Read the model definition and answer for the solid it produces. Units are mm, in the model's axes. Give positions to 0.01 mm unless a question says otherwise; leave off trailing zeros. Order: outer loops, then holes, each group sorted by start corner. A loop starts at its lowest first (then second) coordinate and runs counter-clockwise, first axis right, second up. Notation, with made-up numbers: (82.5, 85.5) - (113.5, 85.5) arc R16 cw to (113.5, 109.5) - close; hole circle Ø8 at (40.25, 10.5). An arc over 180 degrees is marked (long way). Write item = value, one per line.
```python
from build123d import *

# Parameters (mm, degrees)
SKETCH_1_R      = 1.5
SKETCH_1_R_2    = 2
EXTRUDE_1_DEPTH = 3
FILLET_1_R      = 2


with BuildPart() as part:
    # 草图1 → 凸台-拉伸1 (new body)
    with BuildSketch(Plane(origin=(0, 0, 0), x_dir=(1, 0, 0), z_dir=(0, 1, 0))):
        with BuildLine():
            Line((30, -10.5), (20.838488019, -10.5))
            ThreePointArc((20.838488019, -10.5), (19.128387303, -10.801536896), (17.624549971, -11.669777784))
            Line((17.624549971, -11.669777784), (8.432016653, -19.383229101))
            ThreePointArc((8.432016653, -19.383229101), (7.315827683, -20.713451316), (6.721915937, -22.345210428))
            Line((6.721915937, -22.345210428), (2.526313412, -46.139654751))
            Line((2.526313412, -46.139654751), (-18.154649402, -42.49304302))
            Line((-18.154649402, -42.49304302), (-10.267627346, 2.236481777))
            ThreePointArc((-10.267627346, 2.236481777), (-6.847425912, 8.160444431), (-0.419549816, 10.5))
            Line((-0.419549816, 10.5), (30, 10.5))
            Line((30, 10.5), (30, -10.5))
        make_face()
        with Locations(Location((25, 0, 0), (0, 0, 270))):
            Circle(SKETCH_1_R, mode=Mode.SUBTRACT)
        with Locations(Location((10, 0, 0), (0, 0, 270))):
            Circle(SKETCH_1_R, mode=Mode.SUBTRACT)
        with Locations(Location((-6.945927107, -39.39231012, 0), (0, 0, 270))):
            Circle(SKETCH_1_R, mode=Mode.SUBTRACT)
        with Locations(Location((-1.736481777, -9.84807753, 0), (0, 0, 270))):
            Circle(SKETCH_1_R, mode=Mode.SUBTRACT)
        with Locations(Location((10.457132873, -12.46232567, 0), (0, 0, 270))):
            Circle(SKETCH_1_R_2, mode=Mode.SUBTRACT)
    extrude(amount=EXTRUDE_1_DEPTH)

    # 圆角1
    fillet_1_edges = [part.edges().sort_by_distance(p)[0] for p in [
        (2.526313412, 1.5, 46.139654751),
        (-18.154649402, 1.5, 42.49304302),
        (30, 1.5, -10.5),
        (30, 1.5, 10.5),
    ]]
    fillet(fillet_1_edges, radius=FILLET_1_R)


solid = part.part
```
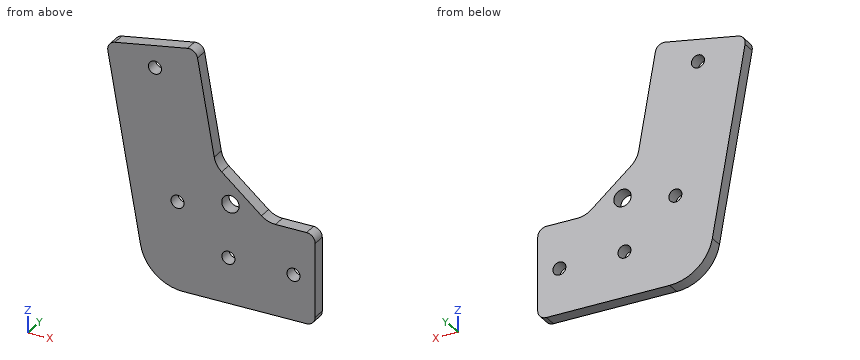
1. Section D-D (z = 0) is taken. Determine the outline of the cut face in (x, y), and give its area (3 significant figures).
Recorded:
outline = (-10.66, 0) - (8.5, 0) - (8.5, 3) - (-10.66, 3) - close; (11.5, 0) - (23.5, 0) - (23.5, 3) - (11.5, 3) - close; (26.5, 0) - (30, 0) - (30, 3) - (26.5, 3) - close
area = 104 mm^2
2. Section B-B (z = 39.5) is taken. Determine the outline of the cut face in (x, y).
Recorded:
outline = (-17.63, 0) - (-8.44, 0) - (-8.44, 3) - (-17.63, 3) - close; (-5.45, 0) - (3.7, 0) - (3.7, 3) - (-5.45, 3) - close
3. Straight lines are drawn through the part: L1, parallel to X at y = 1.5, z = 0; L2, parallel to X at y = 1.9, z = 0.5; L3, parallel to Z at x = 11, y = 0.75. For each, find the intervals that lie inside material, in ascending order. Write a range as [from, to].
Recorded:
L1 = [-10.66, 8.5], [11.5, 23.5], [26.5, 30]
L2 = [-10.75, 8.59], [11.41, 23.59], [26.41, 30]
L3 = [-10.5, -1.12], [1.12, 10.54], [14.39, 17.23]
4. Flat-ended cylindrical pins translate along their axes: pin 1 (1.5 mm diameter, centred on x = -10, y = 2, fed in from -Z); pin 2 (1 mm diameter, centred on y = 2.5, z = 13.5, fed in from +X); pin 3 (1.5 mm diameter, centred on y = 0.5, z = 30.5, fed in from +X). Find the tip coordinate at first contact, or state that the pin passes through.
Recorded:
pin_1 = -5.19
pin_2 = 16.04
pin_3 = 5.42
5. Section C-C (y = 1.25) is taken. Determine the outline of the cut face in (x, z), and give its area (3 significant figures).
Recorded:
outline = (-17.81, 40.52) - (-10.27, -2.24) arc R10 ccw to (-0.42, -10.5) - (28, -10.5) arc R2 ccw to (30, -8.5) - (30, 8.5) arc R2 ccw to (28, 10.5) - (20.84, 10.5) arc R5 cw to (17.62, 11.67) - (8.43, 19.38) arc R5 cw to (6.72, 22.35) - (2.87, 44.17) arc R2 ccw to (0.56, 45.79) - (-16.19, 42.84) arc R2 ccw to start; hole circle Ø3 at (-6.95, 39.39); hole circle Ø3 at (-1.74, 9.85); hole circle Ø4 at (10.46, 12.46); hole circle Ø3 at (10, 0); hole circle Ø3 at (25, 0)
area = 1,570 mm^2
6. Section A-A (x = 25) is taken. Determine the outline of the cut face in (y, z), and give its area (3 significant figures).
Recorded:
outline = (0, -10.5) - (3, -10.5) - (3, -1.5) - (0, -1.5) - close; (0, 1.5) - (3, 1.5) - (3, 10.5) - (0, 10.5) - close
area = 54.0 mm^2
